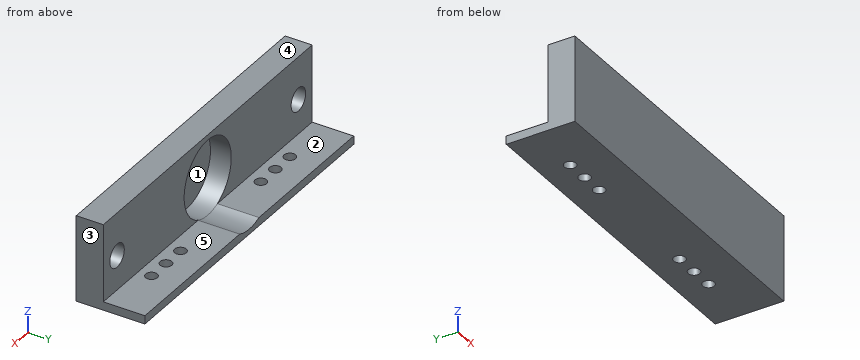
```python
from build123d import *

# Parameters (mm, degrees)
SKETCH1_W           = 102.39
SKETCH1_H           = 26.19
BOSS_EXTRUDE1_DEPTH = 1.905
SKETCH2_W           = 102.39
SKETCH2_H           = 26.19
SKETCH2_R           = 11.557
SKETCH2_R_2         = 3.556
BOSS_EXTRUDE3_DEPTH = 6.35
BOSS_EXTRUDE4_DEPTH = 12.7
CUT_EXTRUDE1_REACH  = 63.204
SKETCH4_R           = 1.778


with BuildPart() as part:
    # Sketch1 → Boss-Extrude1 (new body)
    with BuildSketch(Plane(origin=(0, 0, 0), x_dir=(1, 0, 0), z_dir=(0, 1, 0))):
        Rectangle(SKETCH1_W, SKETCH1_H)
    extrude(amount=BOSS_EXTRUDE1_DEPTH)

    # Sketch2 → Boss-Extrude3 (add)
    with BuildSketch(Plane(origin=(0, 1.905, 0), x_dir=(1, 0, 0), z_dir=(0, 1, 0))):
        Rectangle(SKETCH2_W, SKETCH2_H)
        with Locations(Location((0, 0, 0), (0, 0, 270))):
            Circle(SKETCH2_R, mode=Mode.SUBTRACT)
        with Locations(Location((-44.45, 0, 0), (0, 0, 270))):
            Circle(SKETCH2_R_2, mode=Mode.SUBTRACT)
        with Locations(Location((44.45, 0, 0), (0, 0, 270))):
            Circle(SKETCH2_R_2, mode=Mode.SUBTRACT)
    extrude(amount=BOSS_EXTRUDE3_DEPTH)

    # Sketch3 → Boss-Extrude4 (add)
    with BuildSketch(Plane(origin=(0, 8.255, 0), x_dir=(1, 0, 0), z_dir=(0, 1, 0))):
        with BuildLine():
            Line((-51.195, 13.095), (51.195, 13.095))
            Line((51.195, 13.095), (51.195, 10.555))
            Line((51.195, 10.555), (4.707039834, 10.555))
            ThreePointArc((4.707039834, 10.555), (0, 11.557), (-4.707039834, 10.555))
            Line((-4.707039834, 10.555), (-51.195, 10.555))
            Line((-51.195, 10.555), (-51.195, 13.095))
        make_face()
    extrude(amount=BOSS_EXTRUDE4_DEPTH)

    # Sketch4 → Cut-Extrude1 (cut, up to next)
    with BuildSketch(Plane(origin=(0, 0, -13.095), x_dir=(-1, 0, 0), z_dir=(0, 0, -1)), mode=Mode.PRIVATE) as cut_extrude1_sk1:
        with Locations((33.923, 12.211)):
            Circle(SKETCH4_R)
    cut_extrude1_tool1 = extrude(cut_extrude1_sk1.sketch, amount=-CUT_EXTRUDE1_REACH, mode=Mode.PRIVATE) & part.part
    # Sketch4 → Cut-Extrude1 (cut, up to next)
    with BuildSketch(Plane(origin=(0, 0, -13.095), x_dir=(-1, 0, 0), z_dir=(0, 0, -1)), mode=Mode.PRIVATE) as cut_extrude1_sk2:
        with Locations((26.811, 12.211)):
            Circle(SKETCH4_R)
    cut_extrude1_tool2 = extrude(cut_extrude1_sk2.sketch, amount=-CUT_EXTRUDE1_REACH, mode=Mode.PRIVATE) & part.part
    # Sketch4 → Cut-Extrude1 (cut, up to next)
    with BuildSketch(Plane(origin=(0, 0, -13.095), x_dir=(-1, 0, 0), z_dir=(0, 0, -1)), mode=Mode.PRIVATE) as cut_extrude1_sk3:
        with Locations((19.699, 12.211)):
            Circle(SKETCH4_R)
    cut_extrude1_tool3 = extrude(cut_extrude1_sk3.sketch, amount=-CUT_EXTRUDE1_REACH, mode=Mode.PRIVATE) & part.part
    # Sketch4 → Cut-Extrude1 (cut, up to next)
    with BuildSketch(Plane(origin=(0, 0, -13.095), x_dir=(-1, 0, 0), z_dir=(0, 0, -1)), mode=Mode.PRIVATE) as cut_extrude1_sk4:
        with Locations((-33.923, 12.211)):
            Circle(SKETCH4_R)
    cut_extrude1_tool4 = extrude(cut_extrude1_sk4.sketch, amount=-CUT_EXTRUDE1_REACH, mode=Mode.PRIVATE) & part.part
    # Sketch4 → Cut-Extrude1 (cut, up to next)
    with BuildSketch(Plane(origin=(0, 0, -13.095), x_dir=(-1, 0, 0), z_dir=(0, 0, -1)), mode=Mode.PRIVATE) as cut_extrude1_sk5:
        with Locations((-26.811, 12.211)):
            Circle(SKETCH4_R)
    cut_extrude1_tool5 = extrude(cut_extrude1_sk5.sketch, amount=-CUT_EXTRUDE1_REACH, mode=Mode.PRIVATE) & part.part
    # Sketch4 → Cut-Extrude1 (cut, up to next)
    with BuildSketch(Plane(origin=(0, 0, -13.095), x_dir=(-1, 0, 0), z_dir=(0, 0, -1)), mode=Mode.PRIVATE) as cut_extrude1_sk6:
        with Locations((-19.699, 12.211)):
            Circle(SKETCH4_R)
    cut_extrude1_tool6 = extrude(cut_extrude1_sk6.sketch, amount=-CUT_EXTRUDE1_REACH, mode=Mode.PRIVATE) & part.part
    add(cut_extrude1_tool1.solids().sort_by_distance((-33.923, 12.211, -13.095))[0], mode=Mode.SUBTRACT)
    add(cut_extrude1_tool2.solids().sort_by_distance((-26.811, 12.211, -13.095))[0], mode=Mode.SUBTRACT)
    add(cut_extrude1_tool3.solids().sort_by_distance((-19.699, 12.211, -13.095))[0], mode=Mode.SUBTRACT)
    add(cut_extrude1_tool4.solids().sort_by_distance((33.923, 12.211, -13.095))[0], mode=Mode.SUBTRACT)
    add(cut_extrude1_tool5.solids().sort_by_distance((26.811, 12.211, -13.095))[0], mode=Mode.SUBTRACT)
    add(cut_extrude1_tool6.solids().sort_by_distance((19.699, 12.211, -13.095))[0], mode=Mode.SUBTRACT)


solid = part.part
```
For this review, take the finished solid that the model builds, in its own axes (mm). Face numbers are marked on the shaded views. A direction names the side the tool comes from. Coordinates: 2 decimals unless noted, no trailing zeros. Write each loop counter-clockwise with the first axis right and the second up, starting at its lowest first coordinate (ties: lowest second). Pieces come first, ordered by that corner, then holes. Notation, with made-up numbers: (-3.5, -37.75) - (35.5, -37.75) arc R21 ccw to (35.5, -5.75) - close; hole circle Ø1 at (38.25, 63.5). An arc over 180 degrees is marked (long way). Put each result on its own line as item: value.
1. Add section D-D, the plane z = 8.75. Give the boundary of the cut face in (x, y) (3 decimals), then the cut area to 3 significant figures.
Values found:
outline: (-51.195, 0) - (51.195, 0) - (51.195, 8.255) - (7.55, 8.255) - (7.55, 1.905) - (-7.55, 1.905) - (-7.55, 8.255) - (-51.195, 8.255) - close
area: 749 mm²
2. Add section A-A, the plane x = -27. Give the boundary of the cut face in (y, z) (3 decimals).
Values found:
outline: (0, -13.095) - (10.443, -13.095) - (10.443, -10.555) - (8.255, -10.555) - (8.255, 13.095) - (0, 13.095) - close; (13.979, -13.095) - (20.955, -13.095) - (20.955, -10.555) - (13.979, -10.555) - close
3. Add section C-C, the plane x = 0. Give the boundary of the cut face in (y, z) (3 decimals).
Values found:
outline: (0, -13.095) - (20.955, -13.095) - (20.955, -11.557) - (1.905, -11.557) - (1.905, 11.557) - (8.255, 11.557) - (8.255, 13.095) - (0, 13.095) - close
4. Machinability: for the marked faces 4 and 5, which of the approach directions +Z, -Z, +X, -X, +Y, -Y give a long, thin tool a straight path to every point of the face, cutting with its end or side? Answer none if there is none.
Values found:
face 4: +Z, +X, -X, +Y, -Y
face 5: +Z, +X, -X, +Y
5. Add section B-B, the plane y = 19. Give the boundary of the cut face in (x, z) (3 decimals), then the cut area to 3 significant figures.
Values found:
outline: (-51.195, -13.095) - (51.195, -13.095) - (51.195, -10.555) - (4.707, -10.555) arc R11.557 cw to (-4.707, -10.555) - (-51.195, -10.555) - close
area: 254 mm²
6. For pin 1 (4 mm diameter, centred on x = 33.5, y = 15.5, fed in from +Z) (3 decimals); pin 2 (8 mm diameter, centred on x = 44.45, z = 0, fed in from +Y) (3 decimals); pin 3 (5.5 mm diameter, centred on x = -44.45, z = 0, fed in from +Y) (3 decimals), all flat-tipped, find the tip position at first contact; note any pin that passes through.
Values found:
pin 1: z = -10.555
pin 2: y = 8.255
pin 3: y = 1.905
7. Mouldability with a two-part tool opening along X and no side actions: class the marked faces 1, 2 and 3 as released by +X, released by -X, zero draft, split by the parting line, or undercut.
Values found:
face 1: undercut
face 2: zero draft
face 3: released by +X
8. Wall thickness on probe 1 along X at (y, z) = (5.25, 0) (3 decimals); probe 2 along Y at (x, z) = (-23, 11) (3 decimals); probe 3 along Z at (x, y) = (30, 11.25) (3 decimals): over which ranges is each line inside the solid? List them lowest first.
Values found:
probe 1: -51.195 to -48.006, -40.894 to -11.557, 11.557 to 40.894, 48.006 to 51.195
probe 2: 0 to 8.255
probe 3: -13.095 to -10.555
